Read the model definition and answer for the solid it produces. Units are mm, in the model's axes. Round coordinates to 2 decimals unless told otherwise and drop trailing zeros. Loops run counter-clockwise (first coordinate to the right, second up) from the corner with the lowest first, then second, coordinate; pieces in that order, holes last. Notation, with made-up numbers: (16, 61.25) -> (30, 61.25) arc R7 ccw to (30, 67.25) -> close; hole circle Ø2 at (-17.5, 45). An arc over 180 degrees is marked (long way). Put each result on its own line as item: value.
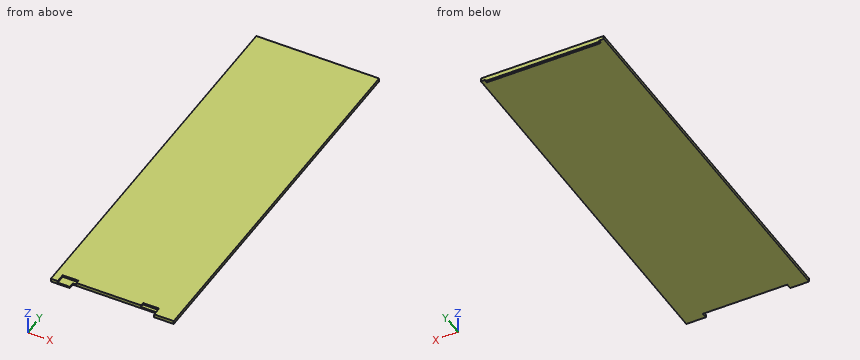
from build123d import *

# Parameters (mm, degrees)
SKETCH1_W           = 108
SKETCH1_H           = 334
BOSS_EXTRUDE1_DEPTH = 2.921
SKETCH2_W           = 74.2
SKETCH2_H           = 4.75075517
CUT_EXTRUDE1_DEPTH  = 176.537837064
SKETCH3_W           = 14
SKETCH3_H           = 1.608195067
CUT_EXTRUDE2_DEPTH  = 8
SKETCH4_W           = 100
SKETCH4_H           = 1.25
BOSS_EXTRUDE2_DEPTH = 2


with BuildPart() as part:
    # Sketch1 → Boss-Extrude1 (new body)
    with BuildSketch(Plane.XY):
        Rectangle(SKETCH1_W, SKETCH1_H)
    extrude(amount=BOSS_EXTRUDE1_DEPTH)

    # Sketch2 → Cut-Extrude1 (cut, through all)
    with BuildSketch(Plane.XY.offset(2.921)):
        with Locations((-0.22, -164.624622415)):
            Rectangle(SKETCH2_W, SKETCH2_H)
    extrude(amount=-CUT_EXTRUDE1_DEPTH, mode=Mode.SUBTRACT)

    # Sketch3 → Cut-Extrude2 (cut)
    with BuildSketch(Plane.XZ.offset(167)):
        with Locations((29.682997172, 2.116902467)):
            Rectangle(SKETCH3_W, SKETCH3_H)
        with Locations((-41, 2.116902467)):
            Rectangle(SKETCH3_W, SKETCH3_H)
    extrude(amount=-CUT_EXTRUDE2_DEPTH, mode=Mode.SUBTRACT)

    # Sketch4 → Boss-Extrude2 (add)
    with BuildSketch(Plane(origin=(0, 167, 0), x_dir=(1, 0, 0), z_dir=(0, 1, 0))):
        with Locations((0, 0.625)):
            Rectangle(SKETCH4_W, SKETCH4_H)
    extrude(amount=-BOSS_EXTRUDE2_DEPTH)


solid = part.part
Item 1: Find the intervals of material crossed by line 1 along Z through (x, y) = (-2.5, -61); line 2 along Y through (x, z) = (-9, 0.7); line 3 along Y through (x, z) = (-35.5, 2.3), in increasing order.
Derived:
line 1: z = 0 to 2.92
line 2: y = -162.25 to 167
line 3: y = -159 to 167
Item 2: Flat-ended cylindrical pins translate along their axes: pin 1 Ø1.5 at (x, y) = (-42.5, 26.5) entering from -Z; pin 2 Ø1.8 at (x, z) = (31.5, 2.5) entering from -Y; pin 3 Ø2.5 at (x, z) = (-12, 1) entering from -Y; pin 4 Ø3.5 at (x, y) = (29.5, -160.5) entering from +Z. Find the tip coordinate at first contact, or state that the pin passes through.
Derived:
pin 1: stops at z = 0
pin 2: stops at y = -159
pin 3: stops at y = -162.25
pin 4: stops at z = 2.92
Item 3: The part is cut by section C-C (y = 77). Determine the outline of the cut face in (x, z).
Derived:
outline: (-54, 0) -> (54, 0) -> (54, 2.92) -> (-54, 2.92) -> close
Item 4: The part is cut by section A-A (x = -21). Determine the outline of the cut face in (y, z), then the cut area to 3 significant figures.
Derived:
outline: (-162.25, 0) -> (165, 0) -> (165, -1.25) -> (167, -1.25) -> (167, 2.92) -> (-162.25, 2.92) -> close
area: 964 mm^2
Item 5: The part is cut by section B-B (x = 41.5). Determine the outline of the cut face in (y, z).
Derived:
outline: (-167, 0) -> (165, 0) -> (165, -1.25) -> (167, -1.25) -> (167, 2.92) -> (-167, 2.92) -> close
